```python
from build123d import *

# Parameters (mm, degrees)
PAD_DEPTH       = 20
POCKET_DEPTH    = 20
SKETCH002_W     = 29.5
SKETCH002_H     = 8.2
POCKET001_DEPTH = 18
SKETCH003_W     = 16.4
SKETCH003_H     = 7.2
SKETCH003_W_2   = 7.6
POCKET002_DEPTH = 5
SKETCH004_W     = 11.1
SKETCH004_H     = 10
POCKET003_DEPTH = 11.5
SKETCH005_W     = 7
SKETCH005_H     = 20.7519948728
POCKET004_DEPTH = 6
FILLET_R        = 2
FILLET001_R     = 1
FILLET002_R     = 1
SKETCH007_W     = 7
SKETCH007_H     = 14
POCKET005_DEPTH = 7
SKETCH008_W     = 7.75
SKETCH008_H     = 8
POCKET006_DEPTH = 6
SKETCH009_R     = 3.75
PAD001_DEPTH    = 4
SKETCH010_R     = 1.6
POCKET007_DEPTH = 20
SKETCH011_W     = 7.75
SKETCH011_H     = 8
POCKET008_DEPTH = 6
SKETCH012_R     = 3.75
PAD002_DEPTH    = 4
SKETCH013_R     = 1.6
POCKET009_DEPTH = 20


with BuildPart() as part:
    # Sketch → Pad (new body)
    with BuildSketch(Plane.YZ):
        Polygon((-19.7132034356, 22.3894444303), (19.7132034356, 22.3894444303), (42.1026478659, 0), (17.3539105243, -24.7487373415), (-17.3539105243, -24.7487373415), (-42.1026478659, 0), align=None)
    extrude(amount=PAD_DEPTH)

    # Sketch001 (on Face8 of Pad) → Pocket (cut)
    with BuildSketch(Plane.YZ.offset(20)):
        Polygon((-35.031580054, 0), (-17.3539105243, -17.6776695297), (-10, -10.3237590053), (-27.6776695297, 7.3539105243), align=None)
        Polygon((10, -10.3237590053), (27.6776695297, 7.3539105243), (35.031580054, 0), (17.3539105243, -17.6776695297), align=None)
    extrude(amount=-POCKET_DEPTH, mode=Mode.SUBTRACT)

    # Sketch002 (on Face5 of Pocket) → Pocket001 (cut)
    with BuildSketch(Plane.YZ.offset(20)):
        with Locations((0, 10.1032575313)):
            Rectangle(SKETCH002_W, SKETCH002_H)
    extrude(amount=-POCKET001_DEPTH, mode=Mode.SUBTRACT)

    # Sketch003 (on Face21 of Pocket001) → Pocket002 (cut)
    with BuildSketch(Plane.YZ.offset(2)):
        with Locations((-5.775, 10.1032575313)):
            Rectangle(SKETCH003_W, SKETCH003_H)
        with Locations((10.175, 10.1032575313)):
            Rectangle(SKETCH003_W_2, SKETCH003_H)
    extrude(amount=-POCKET002_DEPTH, mode=Mode.SUBTRACT)

    # Sketch004 (on Face5 of Pocket002) → Pocket003 (cut)
    with BuildSketch(Plane.YZ.offset(20)):
        with Locations((0, 1.0032575313)):
            Rectangle(SKETCH004_W, SKETCH004_H)
    extrude(amount=-POCKET003_DEPTH, mode=Mode.SUBTRACT)

    # Sketch005 (on Face5 of Pocket003) → Pocket004 (cut)
    with BuildSketch(Plane.YZ.offset(20)):
        with Locations((0, -14.3727399051)):
            Rectangle(SKETCH005_W, SKETCH005_H)
    extrude(amount=-POCKET004_DEPTH, mode=Mode.SUBTRACT)

    # Fillet
    fillet_edges = [part.edges().sort_by_distance(p)[0] for p in [
        (14, 0, -3.996742),
    ]]
    fillet(fillet_edges, radius=FILLET_R)

    # Fillet001
    fillet001_edges = [part.edges().sort_by_distance(p)[0] for p in [
        (17, -3.5, -3.996742),
    ]]
    fillet(fillet001_edges, radius=FILLET001_R)

    # Fillet002
    fillet002_edges = [part.edges().sort_by_distance(p)[0] for p in [
        (17, 3.5, -3.996742),
    ]]
    fillet(fillet002_edges, radius=FILLET002_R)

    # Sketch007 (on Face9 of Fillet002) → Pocket005 (cut)
    with BuildSketch(Plane.YX.offset(24.7487373415)):
        with Locations((0, 7)):
            Rectangle(SKETCH007_W, SKETCH007_H)
    extrude(amount=-POCKET005_DEPTH, mode=Mode.SUBTRACT)

    # Sketch008 (on Face11 of Pocket005) → Pocket006 (cut)
    with BuildSketch(Plane.YZ.offset(20)):
        with Locations((-18.625, 10.1032575313)):
            Rectangle(SKETCH008_W, SKETCH008_H)
    extrude(amount=-POCKET006_DEPTH, mode=Mode.SUBTRACT)

    # Sketch009 (on Face49 of Pocket006) → Pad001 (join)
    with BuildSketch(Plane.YZ.offset(14)):
        with Locations((-18.5, 10.1032575313)):
            Circle(SKETCH009_R)
    extrude(amount=PAD001_DEPTH)

    # Sketch010 (on Face51 of Pad001) → Pocket007 (cut)
    with BuildSketch(Plane.YZ.offset(18)):
        with Locations((-18.5, 10.1032575313)):
            Circle(SKETCH010_R)
    extrude(amount=-POCKET007_DEPTH, mode=Mode.SUBTRACT)

    # Sketch011 (on Face11 of Pocket007) → Pocket008 (cut)
    with BuildSketch(Plane.YZ.offset(20)):
        with Locations((18.625, 10.1032575313)):
            Rectangle(SKETCH011_W, SKETCH011_H)
    extrude(amount=-POCKET008_DEPTH, mode=Mode.SUBTRACT)

    # Sketch012 (on Face54 of Pocket008) → Pad002 (join)
    with BuildSketch(Plane.YZ.offset(14)):
        with Locations((18.5, 10.1032575313)):
            Circle(SKETCH012_R)
    extrude(amount=PAD002_DEPTH)

    # Sketch013 (on Face58 of Pad002) → Pocket009 (cut)
    with BuildSketch(Plane.YZ.offset(18)):
        with Locations((18.5, 10.1032575313)):
            Circle(SKETCH013_R)
    extrude(amount=-POCKET009_DEPTH, mode=Mode.SUBTRACT)


solid = part.part
```
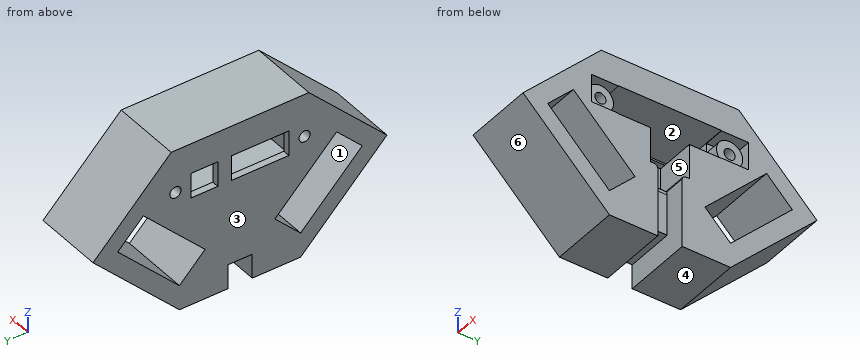
Can you work these out from the model? Positions are in its coordinate system, mm. Face numbers are marked on the shaded views. A direction names the side the tool comes from. Give positions to 0.01 mm unless a question says otherwise; leave off trailing zeros. Order: outer loops, then holes, each group sorted by start corner. A loop starts at its lowest first (then second) coordinate and runs counter-clockwise, first axis right, second up. Notation, with made-up numbers: M 77,-3 L 89,-3 A30 cw 89,32 Z; hole C 54.5,85 d11. An arc over 180 degrees is marked long. One line per item, written item: value.
1) Please list where these lines run through material, in increasing order: line 1 along Z through (x, y) = (7, 9); line 2 along Y through (x, z) = (7, -6.5); line 3 along Z through (x, y) = (8.5, -18.5).
Answer sheet:
line 1: z = -24.75 to 6, 14.2 to 22.39
line 2: y = -35.6 to -28.53, -13.82 to 13.82, 28.53 to 35.6
line 3: z = -23.6 to -16.53, -1.82 to 8.5, 11.7 to 22.39
2) For P1, Ø5, axis at y = -1, z = -0.5, coming from the +X side; P2, Ø10, axis at x = 13, z = -12, coming from the +Y side; P3, Ø1.6, axis at x = 1.5, z = 10.5, coming from the -Y side; P4, Ø6.5, axis at y = 1.5, z = 11, coming from the +X side, each with a flat end and sliding along its axis, tell me the tip position at first contact or that it passes through.
Answer sheet:
P1: stops at x = 8.5
P2: stops at y = 35.1
P3: stops at y = -32.4
P4: stops at x = 20
3) I want a section at A-A, the plane z = -14. List the corners of the cut face in (x, y) for me, plus the area to 3 significant figures.
Answer sheet:
outline: M 0,-28.1 L 20,-28.1 L 20,-21.03 L 0,-21.03 Z; M 0,-13.68 L 20,-13.68 L 20,-3.5 L 14,-3.5 L 14,3.5 L 20,3.5 L 20,13.68 L 0,13.68 Z; M 0,21.03 L 20,21.03 L 20,28.1 L 0,28.1 Z
area: 788 mm^2
4) On a 3-axis mill with a long thin cutter (end or side, diameter ignored), from which of +Z, -Z, +X, -X, +Y, -Y can I reach the whole of each face in a straight line? I mean the marked faces 1, 2 and 3. Say none if no direction works.
Answer sheet:
face 1: +X, -X
face 2: +X
face 3: +Z, -Z, -X, +Y, -Y
5) I want a section at C-C, the plane x = 10.25. List the corners of the cut face in (y, z) for me.
Answer sheet:
outline: M -42.1,0 L -17.35,-24.75 L -3.5,-24.75 L -3.5,-17.75 L 3.5,-17.75 L 3.5,-24.75 L 17.35,-24.75 L 42.1,0 L 19.71,22.39 L -19.71,22.39 Z; hole M -35.03,0 L -17.35,-17.68 L -10,-10.32 L -27.68,7.35 Z; hole C -18.5,10.1 d3.2; hole M -14.75,6 L -5.55,6 L -5.55,-4 L 5.55,-4 L 5.55,6 L 14.75,6 L 14.75,14.2 L -14.75,14.2 Z; hole M 10,-10.32 L 17.35,-17.68 L 35.03,0 L 27.68,7.35 Z; hole C 18.5,10.1 d3.2
6) I want a section at B-B, the plane y = -18.5. List the corners of the cut face in (x, z) for me, plus the area to 3 significant figures.
Answer sheet:
outline: M 0,-23.6 L 20,-23.6 L 20,-16.53 L 0,-16.53 Z; M 0,-1.82 L 20,-1.82 L 20,6.1 L 14,6.1 L 14,6.35 L 18,6.35 L 18,8.5 L 0,8.5 Z; M 0,11.7 L 18,11.7 L 18,13.85 L 14,13.85 L 14,14.1 L 20,14.1 L 20,22.39 L 0,22.39 Z
area: 550 mm^2
7) We'd pull the mould along Y, two halves only. Please class the marked faces 4, 5 and 6: released by +Y, released by -Y, zero draft, split by the parting line, or undercut.
Answer sheet:
face 4: zero draft
face 5: undercut
face 6: released by -Y
8) I want a section at D-D, the plane y = -32.5. List the corners of the cut face in (x, z) for me.
Answer sheet:
outline: M 0,-9.6 L 20,-9.6 L 20,-2.53 L 0,-2.53 Z; M 0,2.53 L 20,2.53 L 20,9.6 L 0,9.6 Z
